The drawing under review shows one solid part. Ordinate dimensions are in mm from its lowest x, y, z. Give positions to 0.01 mm unless a question says otherwise; leave off trailing zeros. Write each loop counter-clockwise with the first axis right and the second up, starting at its lowest first coordinate (ties: lowest second). Pieces come first, ordered by that corner, then holes. Notation, with made-up numbers: (49, 51) - (97, 51) arc R20 cw to (97, 86) - close; hole circle Ø10 at (11.5, 47). An arc over 180 degrees is marked (long way). Write item = value, one per line.
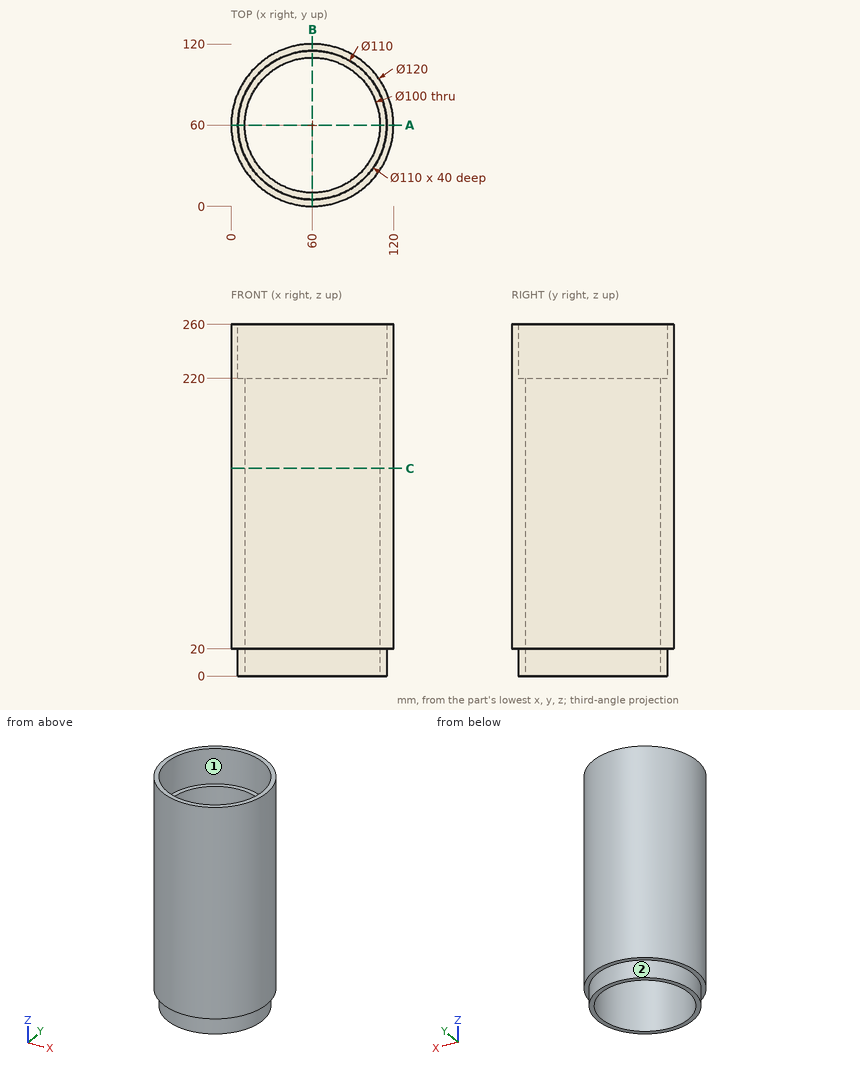
1. For line 1 (Y direction, x = 60, z = 67); line 2 (X direction, y = 61, z = 125.5); line 3 (Y direction, x = 60, z = 241), list the stretches that pass through material, from the lowest coordinate up. Write a range as from..to.
Findings below:
line_1 = 0..10, 110..120
line_2 = 0.01..10.01, 109.99..119.99
line_3 = 0..5, 115..120
2. Insertion check: P1, Ø6, axis at y = 80, z = 91.5, coming from the -X side; P2, Ø1.5, axis at x = 77, z = 41, coming from the -Y side; P3, Ø8, axis at x = 98.5, y = 91.5, coming from the +Z side. Each pin has a flat end and moves straight along its axis. Give the tip position at first contact, or say it passes through.
Findings below:
P1 = 2.46
P2 = 2.24
P3 = 220
3. Take a section at C-C on z = 153.5. Give the boundary of the cut face in (x, y), and give its area (3 significant figures).
Findings below:
outline = circle Ø120 at (60, 60); hole circle Ø100 at (60, 60)
area = 3,460 mm²
4. Take a section at A-A on y = 60. Give the boundary of the cut face in (x, z).
Findings below:
outline = (0, 20) - (5, 20) - (5, 0) - (10, 0) - (10, 220) - (5, 220) - (5, 260) - (0, 260) - close; (110, 0) - (115, 0) - (115, 20) - (120, 20) - (120, 260) - (115, 260) - (115, 220) - (110, 220) - close
5. Draft analysis for pull direction Y (two halves, no side actions). For the marked faces 1 and 2, state which applies: +Y half, -Y half, draft (parallel to the pull), parting line (faces both ways), or undercut.
Findings below:
face_1 = undercut
face_2 = parting line
